Could you check a few things on this model? Use its own coordinates, in mm. A direction names the side the tool comes from. Coordinates: 2 decimals unless noted, no trailing zeros. Write each loop counter-clockwise with the first axis right and the second up, starting at its lowest first coordinate (ties: lowest second). Pieces come first, ordered by that corner, then holes. Notation, with made-up numbers: M 60.5,14 L 105.5,14 A26 cw 105.5,37 Z; hole C 12.5,-26.75 d1. An arc over 180 degrees is marked long. Answer as CSV lines item,"result". Start each with the question number.
Item 1: On a 3-axis mill with a long thin cutter (end or side, diameter ignored), from which of +Z, -Z, +X, -X, +Y, -Y can I reach the whole of each face in a straight line? I mean faces 1 (the flat face through (-10, 45, -44)), 2 (the flat face through (-48, 4, -1)), 3 (the cylindrical face through (-34.51, 1.5, -45.07)). Say none if no direction works.
Item 2: Suppose I cut it at B-B, the plane y = 52.5. Write out the boundary of the cut face in (x, z).
Item 3: Suppose I cut it at A-A, the plane z = -11. Write out the boundary of the cut face in (x, y), and give its area (3 significant figures).
Item 4: I'm going to push flat-ended pins straight in: P1, Ø2, axis at y = 37, z = 43.5, coming from the +X side; P2, Ø4, axis at y = 48, z = -3, coming from the +X side; P3, Ø12, axis at y = 47.5, z = 15.5, coming from the +X side. Where does each tip first touch, or does it pass through?
Item 5: If I drill on line 1 along Z through (x, y) = (-65, 45.5); line 2 along X through (y, z) = (62, 13.5); line 3 along Y through (x, z) = (-85, -31.5), over which ranges is the centre line in solid material (lowest first)? Write a range as [from, to].
Item 6: Suppose I cut it at D-D, the plane y = 10. Write out the boundary of the cut face in (x, z).
Item 7: Suppose I cut it at C-C, the plane x = -37. Write out the boundary of the cut face in (y, z), and give its area (3 significant figures).
Item 8: We'd pull the mould along Y, two halves only. Please class faces 4 (the cylindrical face through (-88.59, 48.1, 34.68)), 5 (the flat face through (-5, 45, 45)), 6 (the flat face through (-98, 90, 0)): +Y half, -Y half, draft (parallel to the pull), parting line (faces both ways), or undercut.
```python
from build123d import *

# Parameters (mm, degrees)
SKETCH_1_W           = 100
SKETCH_1_H           = 93
EXTRUDE_1_DEPTH      = 90
FILLET_8_R           = 30
FILLET_9_R           = 5
SHELL_4_T            = -4
CUT_EXTRUDE_16_DEPTH = 10
FILLET_12_R          = 0.5


with BuildPart() as part:
    # 草圖1 → 填料-伸長1 (new body)
    with BuildSketch(Plane(origin=(0, 0, 0), x_dir=(1, 0, 0), z_dir=(0, 1, 0))):
        with Locations((-50, 0)):
            Rectangle(SKETCH_1_W, SKETCH_1_H)
    extrude(amount=EXTRUDE_1_DEPTH)

    # 圓角8
    fillet_8_edges = [part.edges().sort_by_distance(p)[0] for p in [
        (-100, 45, 46.5),
        (-100, 45, -46.5),
    ]]
    fillet(fillet_8_edges, radius=FILLET_8_R)

    # 圓角9
    fillet_9_edges = [part.edges().sort_by_distance(p)[0] for p in [
        (-100, 0, 0),
        (-35, 0, 46.5),
        (-91.213203436, 0, 37.713203436),
        (-91.213203436, 0, -37.713203436),
        (-35, 0, -46.5),
    ]]
    fillet(fillet_9_edges, radius=FILLET_9_R)

    # 薄殼4
    shell_4_openings = [part.faces().sort_by_distance(p)[0] for p in [
        (-48.123603577, 90, 0),
        (0, 45.056329123, 0),
    ]]
    offset(amount=SHELL_4_T, openings=shell_4_openings, kind=Kind.INTERSECTION)

    # 草圖21 → 除料-伸長16 (cut)
    with BuildSketch(Plane(origin=(0, 0, 0), x_dir=(0, 0, -1), z_dir=(1, 0, 0))):
        Polygon((-42.5, 60), (42.5, 60), (45, 62.5), (45, 27.5), (42.5, 30), (15, 30), (15, 4), (17.5, 1.5), (-17.5, 1.5), (-15, 4), (-15, 30), (-42.5, 30), (-45, 27.5), (-45, 62.5), align=None)
    extrude(amount=-CUT_EXTRUDE_16_DEPTH, mode=Mode.SUBTRACT)

    # 圓角12
    fillet_12_edges = [part.edges().sort_by_distance(p)[0] for p in [
        (-5, 60, -42.5),
        (-5, 62.5, -45),
        (-5, 27.5, -45),
        (-5, 30, -42.5),
        (-5, 4, -15),
        (-5, 1.5, -17.5),
        (-5, 1.5, 17.5),
        (-5, 4, 15),
        (-5, 30, 42.5),
        (-5, 27.5, 45),
        (-5, 62.5, 45),
        (-5, 60, 42.5),
    ]]
    fillet(fillet_12_edges, radius=FILLET_12_R)


solid = part.part
```
Ans:
1,face 1,"+X"
1,face 2,"+X, +Y"
1,face 3,"-Z, +X, -X, -Y"
2,outline,"M -100,-16.5 A30 ccw -70,-46.5 L 0,-46.5 L 0,-45 L -10,-45 L -10,-42.5 L -70,-42.5 A26 cw -96,-16.5 L -96,16.5 A26 cw -70,42.5 L -10,42.5 L -10,45 L 0,45 L 0,46.5 L -70,46.5 A30 ccw -100,16.5 Z"
3,outline,"M -100,5 A5 ccw -95,0 L 0,0 L 0,1.5 L -10,1.5 L -10,4 L -95,4 A1 cw -96,5 L -96,90 L -100,90 Z"
3,area,"714 mm^2"
4,P1,"stops at x = -10"
4,P2,"stops at x = -96"
4,P3,"stops at x = -95.51"
5,line 1,"z = [-46.5, -42.5], [42.5, 46.5]"
5,line 2,"x = [-100, -96]"
5,line 3,"y = [0, 4]"
6,outline,"M -100,-16.5 A30 ccw -70,-46.5 L 0,-46.5 L 0,-42.5 L -70,-42.5 A26 cw -96,-16.5 L -96,16.5 A26 cw -70,42.5 L 0,42.5 L 0,46.5 L -70,46.5 A30 ccw -100,16.5 Z"
7,outline,"M 0,-41.5 A5 ccw 5,-46.5 L 90,-46.5 L 90,-42.5 L 5,-42.5 A1 cw 4,-41.5 L 4,41.5 A1 cw 5,42.5 L 90,42.5 L 90,46.5 L 5,46.5 A5 ccw 0,41.5 Z"
7,area,"1,050 mm^2"
8,face 4,"draft"
8,face 5,"undercut"
8,face 6,"+Y half"
